Work out the finished part from the listing and answer in its coordinate system (mm). A direction names the side the tool comes from. Coordinates: 2 decimals unless noted, no trailing zeros. Order: outer loops, then holes, each group sorted by start corner. A loop starts at its lowest first (then second) coordinate and runs counter-clockwise, first axis right, second up. Notation, with made-up numbers: M 68,1 L 102,1 A24 cw 102,31 Z; hole C -25.5,56 d2. An arc over 180 degrees is marked long. Answer in a Markdown table with one row per item. Add a question column.
Item 1: The part is cut by section B-B (x = 3). Write down the section's boundary in (y, z).
Item 2: Flat-ended cylindrical pins translate along their axes: pin 1 Ø0.9 at (x, y) = (-3.5, 0.5) entering from +Z; pin 2 Ø3 at (x, y) = (0.5, -2.5) entering from +Z; pin 3 Ø1.5 at (x, z) = (2.5, 3) entering from +Y; pin 4 Ø1.5 at (x, y) = (5.5, 2) entering from +Z. Find the tip coordinate at first contact, or state that the pin passes through.
Item 3: The mould has two halves that part along Y. Classify faces 4 (the face through (8, 0, 0)), 5 (the face through (-3, 0, -1.5)), 6 (the face through (4, 2, 0)): released by +Y, released by -Y, zero draft, split by the parting line, or undercut.
Item 4: Which of the six approach directions +Z, -Z, +X, -X, +Y, -Y give full straight-line access (tool end or side, diameter ignored) to faces 1 (the face through (0, 2, -2)), 2 (the face through (-3.014, 1.293, 0.76)), 3 (the face through (-4, 1.3, 1.3))?
Item 5: The part is cut by section C-C (x = -0.5). Write down the section's boundary in (y, z), then the cut area to 3 significant figures.
Item 6: Consider line 1 (X direction, y = 0.75, z = -1.25); line 2 (Z direction, x = 3.75, y = 1); line 3 (Y direction, x = 4, z = 0). Determine where each line is inside the solid, lowest interval first. Write a range as from..to.
Item 7: The part is cut by section A-A (y = 0). Write down the section's boundary in (x, z).
from build123d import *

# Parameters (mm, degrees)
CUT_EXTRUDE1_DEPTH = 2


with BuildPart() as part:
    # Sketch1 → Revolve1 (revolve)
    with BuildSketch(Plane.XY, mode=Mode.PRIVATE) as revolve1_sk:
        Polygon((-4, 0), (8, 0), (8, -1.5705), (7.5705, -2), (0, -2), (0, -3.5), (-3.6, -3.5), (-4, -3.1), align=None)
    revolve(revolve1_sk.sketch.rotate(Axis((-4.6, 0, 0), (1, 0, 0)), 270), axis=Axis((-4.6, 0, 0), (1, 0, 0)))

    # Sketch2 → Cut-Extrude1 (cut)
    with BuildSketch(Plane.ZY.offset(4)):
        Polygon((0, 1.732050808), (-1.5, 0.866025404), (-1.5, -0.866025404), (0, -1.732050808), (1.5, -0.866025404), (1.5, 0.866025404), align=None)
    extrude(amount=-CUT_EXTRUDE1_DEPTH, mode=Mode.SUBTRACT)


solid = part.part
Reply:
| question | item | result |
|---|---|---|
| 1 | outline | C 0,0 d4 |
| 2 | pin 1 | stops at z = 3.5 |
| 2 | pin 2 | stops at z = 3.33 |
| 2 | pin 3 | passes through |
| 2 | pin 4 | stops at z = 1.56 |
| 3 | face 4 | zero draft |
| 3 | face 5 | undercut |
| 3 | face 6 | split by the parting line |
| 4 | face 1 | +X |
| 4 | face 2 | -X |
| 4 | face 3 | +Z, -Z, -X, +Y, -Y |
| 5 | outline | C 0,0 d7 |
| 5 | area | 38.5 mm2 |
| 6 | line 1 | x = -2..8 |
| 6 | line 2 | z = -1.73..1.73 |
| 6 | line 3 | y = -2..2 |
| 7 | outline | M -4,-3.1 L -3.6,-3.5 L 0,-3.5 L 0,-2 L 7.57,-2 L 8,-1.57 L 8,1.57 L 7.57,2 L 0,2 L 0,3.5 L -3.6,3.5 L -4,3.1 L -4,1.5 L -2,1.5 L -2,-1.5 L -4,-1.5 Z |
